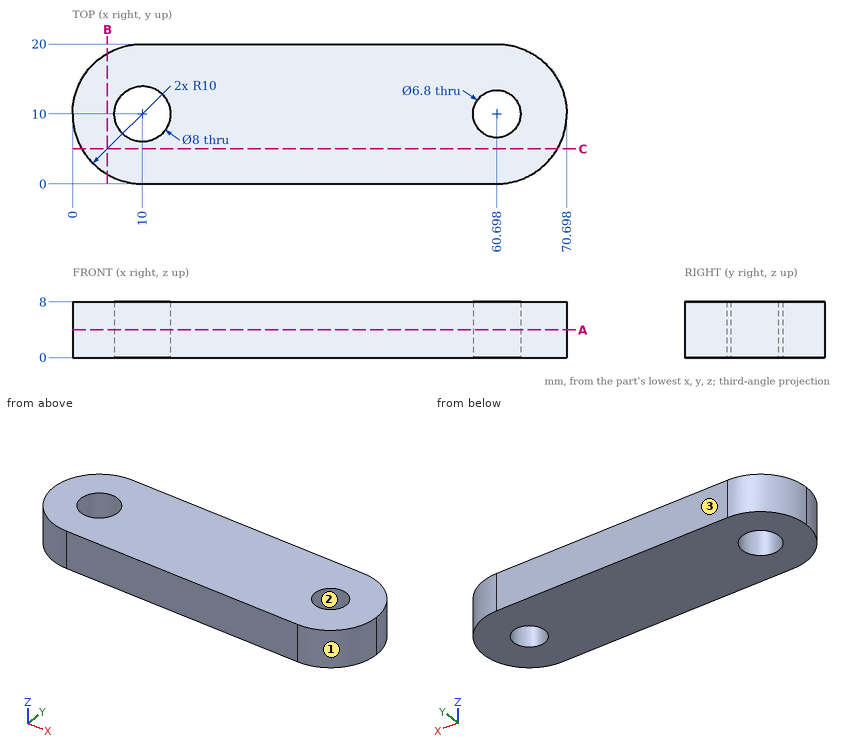
Print and shaded views of the part. All mm, measured from the part's lowest x, y and z. Round coordinates to 2 decimals unless told otherwise and drop trailing zeros. Write each loop counter-clockwise with the first axis right and the second up, starting at its lowest first coordinate (ties: lowest second). Pieces come first, ordered by that corner, then holes. Notation, with made-up numbers: (46, 68) - (58, 68) arc R11 ccw to (58, 77) - close; hole circle Ø7 at (9.5, 88). An arc over 180 degrees is marked (long way). One line per item, written item: value.
(1) Cut at A-A, the plane z = 4. Give the number of separate pieces and of enclosed holes in the cut face, plus the area to 3 significant figures.
Values follow:
separate pieces: 1
enclosed holes: 2
area: 1,240 mm²
(2) Cut at C-C, the plane y = 5. Give the cut face in (x, z), plus the area to 3 significant figures.
Values follow:
outline: (1.34, 0) - (69.36, 0) - (69.36, 8) - (1.34, 8) - close
area: 544 mm²
(3) Drop flat-ended pins along their axis: P1, Ø3, axis at y = 7.5, z = 1.5, coming from the -X side; P2, Ø3, axis at y = 16.5, z = 2, coming from the -X side; P3, Ø3, axis at y = 15, z = 4, coming from the +X side. Give the stop position or say it passes through.
Values follow:
P1: stops at x = 0.05
P2: stops at x = 1.34
P3: stops at x = 70.07
(4) Cut at B-B, the plane x = 5. Give the cut face in (y, z).
Values follow:
outline: (1.34, 0) - (18.66, 0) - (18.66, 8) - (1.34, 8) - close
(5) Wall check: probe 1 along Y at (x, z) = (10, 3.5); probe 2 along X at (y, z) = (11, 3.25); probe 3 along X at (y, z) = (8.75, 1.5). Give the ranges that are in metal, low to high.
Values follow:
probe 1: y = 0 to 6, 14 to 20
probe 2: x = 0.05 to 6.13, 13.87 to 57.45, 63.95 to 70.65
probe 3: x = 0.08 to 6.2, 13.8 to 57.54, 63.86 to 70.62
(6) Two-plate mould, pull along X, no slides. Class the marked faces 1, 2 and 3: pulls with the +X half, pulls with the -X half, needs draft (parallel to the pull), parting line crosses it, or undercut.
Values follow:
face 1: pulls with the +X half
face 2: undercut
face 3: needs draft
